CAD build for the part. Positions are in the model's coordinates, mm. A direction names the side the tool comes from. Coordinates: 2 decimals unless noted, no trailing zeros. Order: outer loops, then holes, each group sorted by start corner. A loop starts at its lowest first (then second) coordinate and runs counter-clockwise, first axis right, second up. Notation, with made-up numbers: (-1.5, 28.5) - (33.5, 28.5) arc R27 cw to (33.5, 65.5) - close; hole circle Ø7 at (44.5, 49). An arc over 180 degrees is marked (long way). Return JSON: item names as keys, results as strings.
from build123d import *

# Parameters (mm, degrees)
SKETCH1_W           = 13.701960198
SKETCH1_H           = 8.105384906
BOSS_EXTRUDE1_DEPTH = 3
CAVITY1_OUTLINE_W   = 13.701960198
CAVITY1_OUTLINE_H   = 8.105384906
CAVITY1_DEPTH       = 2.5
CUT_EXTRUDE1_DEPTH  = 1.5
FILLET1_R           = 1
FILLET2_R           = 1


with BuildPart() as part:
    # Sketch1 → Boss-Extrude1 (new body)
    with BuildSketch(Plane.XY):
        with Locations((6.850980099, 4.052692453)):
            Rectangle(SKETCH1_W, SKETCH1_H)
    extrude(amount=BOSS_EXTRUDE1_DEPTH)

    # Cavity1: read off the stored shape, not the designer's step
    # Cavity1 outline → Cavity1 (cut)
    with BuildSketch(Plane.XY):
        with Locations((6.850980099, 4.052692453)):
            Rectangle(CAVITY1_OUTLINE_W, CAVITY1_OUTLINE_H)
        with BuildLine():
            Line((11.821561481, 4.585876247), (11.821561481, 3.315876247))
            ThreePointArc((11.821561481, 3.315876247), (11.528668262, 2.608769466), (10.821561481, 2.315876247))
            Line((10.821561481, 2.315876247), (4.051561481, 2.315876247))
            ThreePointArc((4.051561481, 2.315876247), (3.3444547, 2.608769466), (3.051561481, 3.315876247))
            Line((3.051561481, 3.315876247), (3.051561481, 4.585876247))
            ThreePointArc((3.051561481, 4.585876247), (3.3444547, 5.292983028), (4.051561481, 5.585876247))
            Line((4.051561481, 5.585876247), (10.821561481, 5.585876247))
            ThreePointArc((10.821561481, 5.585876247), (11.528668262, 5.292983028), (11.821561481, 4.585876247))
        make_face(mode=Mode.SUBTRACT)
    extrude(amount=CAVITY1_DEPTH, mode=Mode.SUBTRACT)

    # Cavity1 2: loft between two sections, ruled curve by curve
    cavity1_2_from = [
        Edge.make_three_point_arc((3.051561481, 3.315876247, 2.2), (3.3444547, 2.608769466, 2.2), (4.051561481, 2.315876247, 2.2)),
        Edge.make_three_point_arc((4.051561481, 5.585876247, 2.2), (3.3444547, 5.292983028, 2.2), (3.051561481, 4.585876247, 2.2)),
        Edge.make_three_point_arc((10.821561481, 2.315876247, 2.2), (11.528668262, 2.608769466, 2.2), (11.821561481, 3.315876247, 2.2)),
        Edge.make_three_point_arc((11.821561481, 4.585876247, 2.2), (11.528668262, 5.292983028, 2.2), (10.821561481, 5.585876247, 2.2)),
        Edge.make_line((3.051561481, 4.585876247, 2.2), (3.051561481, 3.315876247, 2.2)),
        Edge.make_line((4.051561481, 2.315876247, 2.2), (10.821561481, 2.315876247, 2.2)),
        Edge.make_line((4.051561481, 5.585876247, 2.2), (10.821561481, 5.585876247, 2.2)),
        Edge.make_line((11.821561481, 3.315876247, 2.2), (11.821561481, 4.585876247, 2.2)),
    ]
    cavity1_2_to = [
        Edge.make_three_point_arc((2.751561481, 3.315876247, 2.5), (3.132322665, 2.396637431, 2.5), (4.051561481, 2.015876247, 2.5)),
        Edge.make_three_point_arc((4.051561481, 5.885876247, 2.5), (3.132322665, 5.505115063, 2.5), (2.751561481, 4.585876247, 2.5)),
        Edge.make_three_point_arc((10.821561481, 2.015876247, 2.5), (11.740800297, 2.396637431, 2.5), (12.121561481, 3.315876247, 2.5)),
        Edge.make_three_point_arc((12.121561481, 4.585876247, 2.5), (11.740800297, 5.505115063, 2.5), (10.821561481, 5.885876247, 2.5)),
        Edge.make_line((2.751561481, 4.585876247, 2.5), (2.751561481, 3.315876247, 2.5)),
        Edge.make_line((4.051561481, 2.015876247, 2.5), (10.821561481, 2.015876247, 2.5)),
        Edge.make_line((4.051561481, 5.885876247, 2.5), (10.821561481, 5.885876247, 2.5)),
        Edge.make_line((12.121561481, 3.315876247, 2.5), (12.121561481, 4.585876247, 2.5)),
    ]
    cavity1_2 = Solid(Shell([*[Face.make_surface_from_curves(cavity1_2_from[k], cavity1_2_to[k]) for k in range(8)], Face(Wire(cavity1_2_from)), Face(Wire(cavity1_2_to))]))
    add(cavity1_2)

    # Sketch2 → Cut-Extrude1 (cut)
    with BuildSketch(Plane(origin=(0, 0, 0), x_dir=(-1, 0, 0), z_dir=(0, 0, -1))):
        with BuildLine():
            Line((-3.851561481, 3.315876247), (-3.851561481, 4.585876247))
            ThreePointArc((-3.851561481, 4.585876247), (-3.910140125, 4.727297603), (-4.051561481, 4.785876247))
            Line((-4.051561481, 4.785876247), (-10.821561481, 4.785876247))
            ThreePointArc((-10.821561481, 4.785876247), (-10.962982837, 4.727297603), (-11.021561481, 4.585876247))
            Line((-11.021561481, 4.585876247), (-11.021561481, 3.315876247))
            ThreePointArc((-11.021561481, 3.315876247), (-10.962982837, 3.174454891), (-10.821561481, 3.115876247))
            Line((-10.821561481, 3.115876247), (-4.051561481, 3.115876247))
            ThreePointArc((-4.051561481, 3.115876247), (-3.910140125, 3.174454891), (-3.851561481, 3.315876247))
        make_face()
    extrude(amount=-CUT_EXTRUDE1_DEPTH, mode=Mode.SUBTRACT)

    # Fillet1
    fillet1_edges = [part.edges().sort_by_distance(p)[0] for p in [
        (0, 8.105384906, 2.75),
        (13.701960198, 8.105384906, 2.75),
        (13.701960198, 0, 2.75),
        (0, 0, 2.75),
    ]]
    fillet(fillet1_edges, radius=FILLET1_R)

    # Fillet2
    # the kernel refuses this fillet: 1 mm, written as the material it takes off along each edge
    with BuildSketch(Plane(origin=(1, 1, 3), x_dir=(-1, 0, 0), z_dir=(0, 1, 0))) as fillet2_piece_1:
        with BuildLine():
            CenterArc((0.133974596, -1), FILLET2_R, 30, 60)
            Line((0.133974596, 0), (0.133974596, 0.02))
            Line((0.133974596, 0.02), (1, 0.02))
            Line((1, 0.02), (1.02, 0))
            ThreePointArc((1.02, 0), (1.02, -0.25), (1.017320508, -0.49))
            Line((1.017320508, -0.49), (1, -0.5))
        make_face()
    revolve(axis=Axis((1, 1, 3), (0, 0, 1)), revolution_arc=90, mode=Mode.SUBTRACT)
    with BuildSketch(Plane(origin=(0, 7.105384906, 3), x_dir=(0, 0, -1), z_dir=(0, -1, 0)), Plane(origin=(13.701960198, 1, 3), x_dir=(-5.230269550793082e-10, 0, -1.0), z_dir=(0, 1, 0))) as fillet2_piece_2:
        with BuildLine():
            CenterArc((1, 0.866025404), FILLET2_R, 180, 60)
            Line((0, 0.866025404), (-0.02, 0.866025404))
            Line((-0.02, 0.866025404), (-0.02, 0))
            Line((-0.02, 0), (0, -0.02))
            ThreePointArc((0, -0.02), (0.25, -0.02), (0.49, -0.017320508))
            Line((0.49, -0.017320508), (0.5, 0))
        make_face()
    extrude(amount=6.105384906, mode=Mode.SUBTRACT)
    with BuildSketch(Plane(origin=(1, 7.105384906, 3), x_dir=(-1, 0, 0), z_dir=(0, -1, 0))) as fillet2_piece_3:
        with BuildLine():
            CenterArc((0.133974596, 1), FILLET2_R, 270, 60)
            Line((0.133974596, 0), (0.133974596, -0.02))
            Line((0.133974596, -0.02), (1, -0.02))
            Line((1, -0.02), (1.02, 0))
            ThreePointArc((1.02, 0), (1.02, 0.25), (1.017320508, 0.49))
            Line((1.017320508, 0.49), (1, 0.5))
        make_face()
    revolve(axis=Axis((1, 7.105384906, 3), (0, 0, -1)), revolution_arc=90, mode=Mode.SUBTRACT)
    with BuildSketch(Plane(origin=(12.701960198, 8.105384906, 3), x_dir=(0, -2.7725377549357952e-11, -1.0), z_dir=(-1, 0, 0)), Plane(origin=(1, 0, 3), x_dir=(0, 0, -1), z_dir=(1, 0, 0))) as fillet2_piece_4:
        with BuildLine():
            CenterArc((1, 0.866025404), FILLET2_R, 179.999999998, 60)
            Line((0, 0.866025404), (-0.02, 0.866025404))
            Line((-0.02, 0.866025404), (-0.02, 0))
            Line((-0.02, 0), (0, -0.02))
            ThreePointArc((0, -0.02), (0.25, -0.02), (0.49, -0.017320508))
            Line((0.49, -0.017320508), (0.5, 0))
        make_face()
    extrude(amount=11.701960198, mode=Mode.SUBTRACT)
    with BuildSketch(Plane(origin=(12.701960198, 7.105384906, 3), x_dir=(0, 1, 0), z_dir=(-1, 0, 0))) as fillet2_piece_5:
        with BuildLine():
            CenterArc((0.133974596, 1), FILLET2_R, 270, 60)
            Line((0.133974596, 0), (0.133974596, -0.02))
            Line((0.133974596, -0.02), (1, -0.02))
            Line((1, -0.02), (1.02, 0))
            ThreePointArc((1.02, 0), (1.02, 0.25), (1.017320508, 0.49))
            Line((1.017320508, 0.49), (1, 0.5))
        make_face()
    revolve(axis=Axis((12.701960198, 7.105384906, 3), (0, 0, -1)), revolution_arc=90, mode=Mode.SUBTRACT)
    with BuildSketch(Plane(origin=(12.701960198, 1, 3), x_dir=(0, -1, 0), z_dir=(-1, 0, 0))) as fillet2_piece_6:
        with BuildLine():
            CenterArc((0.133974596, -1), FILLET2_R, 30, 60)
            Line((0.133974596, 0), (0.133974596, 0.02))
            Line((0.133974596, 0.02), (1, 0.02))
            Line((1, 0.02), (1.02, 0))
            ThreePointArc((1.02, 0), (1.02, -0.25), (1.017320508, -0.49))
            Line((1.017320508, -0.49), (1, -0.5))
        make_face()
    revolve(axis=Axis((12.701960198, 1, 3), (0, 0, 1)), revolution_arc=90, mode=Mode.SUBTRACT)


solid = part.part
Item 1: Which spindle directions (+Z, -Z, +X, -X, +Y, -Y) get a long thin tool onto all of the face, cutting with end or side? Do faces 5 (the flat face through (3.852, 4, 1)), 6 (the flat face through (3.052, 4, 1)), 7 (the cylindrical face through (3.34, 5.29, 1.08)), 8 (the cylindrical face through (11.52, 5.3, 1.08)), 9 (the flat face through (7, 2.316, 1)). Say none if no direction does.
Findings below:
{"face 5": "-Z", "face 6": "-Z, -X, +Y, -Y", "face 7": "-Z, -X, +Y", "face 8": "-Z, +X, +Y", "face 9": "-Z, +X, -X, -Y"}
Item 2: Mould opens along X. For faces 1 (the flat face through (7, 5.586, 1)), 2 (the flat face through (11.022, 4, 1)), 3 (the flat face through (7, 4.786, 1)), 4 (the cylindrical face through (0.37, 4.1, 2.87)) say: released by +X, released by -X, zero draft, split by the parting line, or undercut.
Findings below:
{"face 1": "zero draft", "face 2": "undercut", "face 3": "undercut", "face 4": "released by -X"}
Item 3: Wall check: L1, parallel to Y at x = 5.5, z = 1.3; L2, parallel to X at y = 3.75, z = 0.35; L3, parallel to Z at x = 7, y = 3.5. Give the ranges that are in metal, low to high. Write a range as [from, to].
Findings below:
{"L1": "y = [2.32, 3.12], [4.79, 5.59]", "L2": "x = [3.05, 3.85], [11.02, 11.82]", "L3": "z = [1.5, 3]"}
Item 4: Band-saw the part on C-C, the plane x = 2. List the corners of the cut face in (y, z).
Findings below:
{"outline": "(0, 2.5) - (8.11, 2.5) arc R1 ccw to (7.24, 3) - (0.87, 3) arc R1 ccw to start"}
Item 5: Band-saw the part on A-A, the plane z = 0.75. List the corners of the cut face in (x, y).
Findings below:
{"outline": "(3.05, 3.32) arc R1 ccw to (4.05, 2.32) - (10.82, 2.32) arc R1 ccw to (11.82, 3.32) - (11.82, 4.59) arc R1 ccw to (10.82, 5.59) - (4.05, 5.59) arc R1 ccw to (3.05, 4.59) - close; hole (3.85, 3.32) arc R0.2 ccw to (4.05, 3.12) - (10.82, 3.12) arc R0.2 ccw to (11.02, 3.32) - (11.02, 4.59) arc R0.2 ccw to (10.82, 4.79) - (4.05, 4.79) arc R0.2 ccw to (3.85, 4.59) - close"}
Item 6: Band-saw the part on B-B, the plane z = 1.8. List the corners of the cut face in (x, y), then the cut area to 3 significant figures.
Findings below:
{"outline": "(3.05, 3.32) arc R1 ccw to (4.05, 2.32) - (10.82, 2.32) arc R1 ccw to (11.82, 3.32) - (11.82, 4.59) arc R1 ccw to (10.82, 5.59) - (4.05, 5.59) arc R1 ccw to (3.05, 4.59) - close", "area": "27.8 mm²"}
Item 7: Drop flat-ended pins along their axis: P1, Ø1, axis at x = 5, y = 7, coming from the -Z side; P2, Ø1.5, axis at y = 3.5, z = 1.5, coming from the +X side; P3, Ø0.5, axis at x = 8, y = 3.5, coming from the -Z side. Give the stop position or say it passes through.
Findings below:
{"P1": "stops at z = 2.5", "P2": "stops at x = 11.87", "P3": "stops at z = 1.5"}
